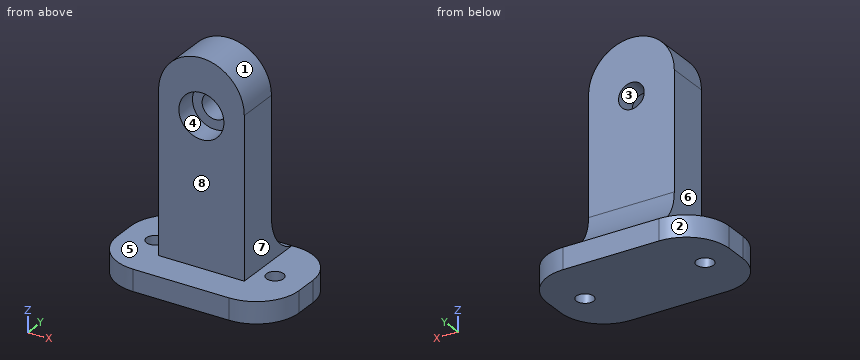
```python
from build123d import *

# Parameters (mm, degrees)
SKETCH1_W           = 42.425590724
SKETCH1_H           = 25
SKETCH1_R           = 2
BOSS_EXTRUDE1_DEPTH = 5
FILLET1_R           = 10
SKETCH2_W           = 20
SKETCH2_H           = 10
BOSS_EXTRUDE2_DEPTH = 47
SKETCH3_R           = 5.25
CUT_EXTRUDE1_DEPTH  = 5
SKETCH4_R           = 3
CUT_EXTRUDE2_DEPTH  = 5
FILLET2_R           = 10


with BuildPart() as part:
    # Sketch1 → Boss-Extrude1 (new body)
    with BuildSketch(Plane.XY):
        Rectangle(SKETCH1_W, SKETCH1_H)
        with Locations((-14, 0)):
            Circle(SKETCH1_R, mode=Mode.SUBTRACT)
        with Locations(Location((14, 0, 0), (0, 0, 180))):
            Circle(SKETCH1_R, mode=Mode.SUBTRACT)
    extrude(amount=BOSS_EXTRUDE1_DEPTH)

    # Fillet1
    fillet1_edges = [part.edges().sort_by_distance(p)[0] for p in [
        (-21.212795362, 12.5, 2.5),
        (21.212795362, 12.5, 2.5),
        (21.212795362, -12.5, 2.5),
        (-21.212795362, -12.5, 2.5),
    ]]
    fillet(fillet1_edges, radius=FILLET1_R)

    # Sketch2 → Boss-Extrude2 (add)
    with BuildSketch(Plane.XY.offset(5)):
        Rectangle(SKETCH2_W, SKETCH2_H)
    extrude(amount=BOSS_EXTRUDE2_DEPTH)

    # Sketch3 → Cut-Extrude1 (cut)
    with BuildSketch(Plane.XZ.offset(5)):
        with Locations((0, 39)):
            Circle(SKETCH3_R)
    extrude(amount=-CUT_EXTRUDE1_DEPTH, mode=Mode.SUBTRACT)

    # Sketch4 → Cut-Extrude2 (cut)
    with BuildSketch(Plane.XZ):
        with Locations((0, 39)):
            Circle(SKETCH4_R)
    extrude(amount=-CUT_EXTRUDE2_DEPTH, mode=Mode.SUBTRACT)

    # Fillet2
    # the kernel refuses this fillet: 10 mm, written as the material it adds along each edge
    with BuildSketch(Plane(origin=(-10, 5, 5), x_dir=(0, 1, 0), z_dir=(1, 0, 0))) as fillet2_piece_1:
        with BuildLine():
            CenterArc((10, 9.682458366), FILLET2_R, 180, 75.522487814)
            Line((0, 9.682458366), (0, 0))
            Line((0, 0), (7.5, 0))
        make_face()
    extrude(amount=20)
    # the kernel refuses this fillet: 10 mm, written as the material it takes off along each edge
    with BuildSketch(Plane(origin=(-10, -30, 52), x_dir=(1, 0, 0), z_dir=(0, 1, 0))) as fillet2_2_piece_1:
        with BuildLine():
            CenterArc((FILLET2_R, FILLET2_R), FILLET2_R, 180, 90)
            Line((0, FILLET2_R), (0, 0))
            Line((0, 0), (FILLET2_R, 0))
        make_face()
    extrude(amount=60, mode=Mode.SUBTRACT)
    with BuildSketch(Plane(origin=(10, 30, 52), x_dir=(0, 0, -1), z_dir=(0, -1, 0))) as fillet2_2_piece_2:
        with BuildLine():
            CenterArc((FILLET2_R, -FILLET2_R), FILLET2_R, 90, 90)
            Line((0, -FILLET2_R), (0, 0))
            Line((0, 0), (FILLET2_R, 0))
        make_face()
    extrude(amount=60, mode=Mode.SUBTRACT)


solid = part.part
```
Here's how the part is built. I have some questions about the finished solid (model axes, mm). Face numbers are marked on the shaded views. A direction names the side the tool comes from. Round coordinates to 2 decimals unless told otherwise and drop trailing zeros. Order: outer loops, then holes, each group sorted by start corner. A loop starts at its lowest first (then second) coordinate and runs counter-clockwise, first axis right, second up. Notation, with made-up numbers: (-14, 46.5) -> (35, 46.5) arc R25 cw to (35, 58.5) -> close; hole circle Ø6 at (-40, 39). An arc over 180 degrees is marked (long way). Use a Markdown table: item, result. Add a question column.
(1) I need wall thicknesses on line 1 along Z through (x, y) = (0, 3.8); line 2 along Z through (x, y) = (-15.5, -9.5); line 3 along Y through (x, z) = (-13.5, 3.5). Which ranges of each line are inside material? Lowest first, please.
(2) Suppose I cut it at D-D, the plane y = 5.75. Please give me the cut outline in (x, z), and give its area (3 significant figures).
(3) For the marked faces 5, 6, 7 and 8, which set-ups out of +Z, -Z, +X, -X, +Y, -Y let a thin tool reach every point of the face, with its end or its side?
(4) If we mould it in two halves opening along Z, with no side actions, what happens to the marked faces 1, 2, 3 and 4? For each: released by +Z, released by -Z, zero draft, split by the parting line, or undercut.
(5) Suppose I cut it at C-C, the plane y = -0.75. Please give me the cut outline in (x, z), and give its area (3 significant figures).
(6) For pin 1 Ø12.5 at (x, y) = (10, -5) entering from +Z; pin 2 Ø1 at (x, z) = (-8, 16.5) entering from -Y; pin 3 Ø3.5 at (x, y) = (-14, 0) entering from +Z; pin 4 Ø22 at (x, z) = (-3, 38.5) entering from +Y, each with a flat end and sliding along its axis, tell me the tip position at first contact or that it passes through.
(7) Suppose I cut it at B-B, the plane x = 0. Please give me the cut outline in (y, z).
(8) Suppose I cut it at A-A, the plane z = 39. Please give me the cut outline in (x, y).
Verdict:
| question | item | result |
|---|---|---|
| 1 | line 1 | 0 to 36, 42 to 52 |
| 1 | line 2 | 0 to 5 |
| 1 | line 3 | -12.23 to -1.94, 1.94 to 12.23 |
| 2 | outline | (-20.67, 0) -> (20.67, 0) -> (20.67, 5) -> (10, 5) -> (10, 10.88) -> (-10, 10.88) -> (-10, 5) -> (-20.67, 5) -> close |
| 2 | area | 324 mm2 |
| 3 | face 5 | +Z, -Y |
| 3 | face 6 | +Z, -X, +Y, -Y |
| 3 | face 7 | +Z, +X, +Y, -Y |
| 3 | face 8 | +Z, +X, -X, -Y |
| 4 | face 1 | released by +Z |
| 4 | face 2 | zero draft |
| 4 | face 3 | undercut |
| 4 | face 4 | undercut |
| 5 | outline | (-21.21, 0) -> (-15.85, 0) -> (-15.85, 5) -> (-21.21, 5) -> close; (-12.15, 0) -> (12.15, 0) -> (12.15, 5) -> (10, 5) -> (10, 42) arc R10 ccw to (-10, 42) -> (-10, 5) -> (-12.15, 5) -> close; (15.85, 0) -> (21.21, 0) -> (21.21, 5) -> (15.85, 5) -> close; hole circle Ø10.5 at (0, 39) |
| 5 | area | 986 mm2 |
| 6 | pin 1 | z = 51.27 |
| 6 | pin 2 | y = -5 |
| 6 | pin 3 | through |
| 6 | pin 4 | y = 5 |
| 7 | outline | (-12.5, 0) -> (12.5, 0) -> (12.5, 5) arc R10 cw to (5, 14.68) -> (5, 36) -> (0, 36) -> (0, 33.75) -> (-5, 33.75) -> (-5, 5) -> (-12.5, 5) -> close; (-5, 44.25) -> (0, 44.25) -> (0, 42) -> (5, 42) -> (5, 52) -> (-5, 52) -> close |
| 8 | outline | (-10, -5) -> (-5.25, -5) -> (-5.25, 0) -> (-3, 0) -> (-3, 5) -> (-10, 5) -> close; (3, 0) -> (5.25, 0) -> (5.25, -5) -> (10, -5) -> (10, 5) -> (3, 5) -> close |
